from build123d import *

# Parameters (mm, degrees)
SKETCH1_R             = 30.5
SKETCH1_R_2           = 28.5
BOSS_EXTRUDE1_DEPTH   = 1.3
BOSS_EXTRUDE1_2_DEPTH = 1.3
BOSS_EXTRUDE1_3_DEPTH = 1.3
BOSS_EXTRUDE1_4_DEPTH = 1.3
SKETCH3_R             = 1
BOSS_EXTRUDE2_DEPTH   = 1.3


with BuildPart() as part:
    # Sketch1 → Boss-Extrude1 (new body)
    with BuildSketch(Plane.XY):
        with Locations((-31.819805153, 31.819805153)):
            Circle(SKETCH1_R)
        with Locations((-31.819805153, 31.819805153)):
            Circle(SKETCH1_R_2, mode=Mode.SUBTRACT)
    extrude(amount=BOSS_EXTRUDE1_DEPTH)



with BuildPart() as body_2:
    # Sketch1 → Boss-Extrude1 2 (new body)
    with BuildSketch(Plane.XY):
        with Locations((31.819805153, 31.819805153)):
            Circle(SKETCH1_R)
        with Locations((31.819805153, 31.819805153)):
            Circle(SKETCH1_R_2, mode=Mode.SUBTRACT)
    extrude(amount=BOSS_EXTRUDE1_2_DEPTH)


with BuildPart() as body_3:
    # Sketch1 → Boss-Extrude1 3 (new body)
    with BuildSketch(Plane.XY):
        with Locations((31.819805153, -31.819805153)):
            Circle(SKETCH1_R)
        with Locations((31.819805153, -31.819805153)):
            Circle(SKETCH1_R_2, mode=Mode.SUBTRACT)
    extrude(amount=BOSS_EXTRUDE1_3_DEPTH)


with BuildPart() as body_4:
    # Sketch1 → Boss-Extrude1 4 (new body)
    with BuildSketch(Plane.XY):
        with Locations((-31.819805153, -31.819805153)):
            Circle(SKETCH1_R)
        with Locations((-31.819805153, -31.819805153)):
            Circle(SKETCH1_R_2, mode=Mode.SUBTRACT)
    extrude(amount=BOSS_EXTRUDE1_4_DEPTH)


with BuildPart() as part_1:
    add(part.part)

    add(body_2.part)  # Boss-Extrude2 merges body 2

    add(body_3.part)  # Boss-Extrude2 merges body 3

    add(body_4.part)  # Boss-Extrude2 merges body 4
    # Sketch3 → Boss-Extrude2 (add)
    with BuildSketch(Plane(origin=(0, 0, 0), x_dir=(-1, 0, 0), z_dir=(0, 0, -1))):
        with BuildLine():
            ThreePointArc((-23.75, 0), (-20.75, -3), (-17.75, 0))
            ThreePointArc((-17.75, 0), (-20.75, 3), (-23.75, 0))
        make_face()
        with Locations((-20.75, 0)):
            Circle(SKETCH3_R, mode=Mode.SUBTRACT)
        with BuildLine():
            ThreePointArc((-14.160081763, -6.952473777), (-16.799552066, -3.912301259), (-17.75, 0))
            ThreePointArc((-17.75, 0), (-20.75, -3), (-23.75, 0))
            ThreePointArc((-23.75, 0), (-24.444680466, -1.473679275), (-26.023521849, -1.875638779))
            ThreePointArc((-26.023521849, -1.875638779), (-19.820237414, -3.779470382), (-14.160081763, -6.952473777))
        make_face()
        with BuildLine():
            ThreePointArc((-23.75, 0), (-20.75, 3), (-17.75, 0))
            ThreePointArc((-17.75, 0), (-16.799552066, 3.912301259), (-14.160081763, 6.952473777))
            ThreePointArc((-14.160081763, 6.952473777), (-19.820237414, 3.779470382), (-26.023521849, 1.875638779))
            ThreePointArc((-26.023521849, 1.875638779), (-24.444680466, 1.473679275), (-23.75, 0))
        make_face()
        with BuildLine():
            add(Edge.make_bspline(
                [(-14.160081763, -6.952473777), (-14.006442935, -7.061581552), (-11.281305453, -8.851296282), (-5.533016891, -10.311083757), (-0.273902085, -10.375), (0, -10.375)],
                knots=[0, 0, 0, 0, 0.05, 0.95, 1, 1, 1, 1], degree=3))
            ThreePointArc((-14.160081763, -6.952473777), (-7.656423025, -13.208492354), (-3.268059498, -21.093770469))
            ThreePointArc((-3.268059498, -21.093770469), (-2.8699742, -17.878412259), (0, -16.375))
            ThreePointArc((0, -16.375), (-3, -13.375), (0, -10.375))
        make_face()
        with BuildLine():
            ThreePointArc((-3.268059498, 21.093770469), (-7.656423025, 13.208492354), (-14.160081763, 6.952473777))
            add(Edge.make_bspline(
                [(-14.160081763, 6.952473777), (-14.006442935, 7.061581552), (-11.281305453, 8.851296282), (-5.533016891, 10.311083757), (-0.273902085, 10.375), (0, 10.375)],
                knots=[0, 0, 0, 0, 0.05, 0.95, 1, 1, 1, 1], degree=3))
            ThreePointArc((0, 10.375), (-3, 13.375), (0, 16.375))
            ThreePointArc((0, 16.375), (-2.8699742, 17.878412259), (-3.268059498, 21.093770469))
        make_face()
        with BuildLine():
            add(Edge.make_bspline(
                [(14.160081763, -6.952473777), (14.006442935, -7.061581552), (11.281305453, -8.851296282), (5.533016891, -10.311083757), (0.273902085, -10.375), (0, -10.375)],
                knots=[0, 0, 0, 0, 0.05, 0.95, 1, 1, 1, 1], degree=3))
            ThreePointArc((0, -10.375), (2.121320344, -11.253679656), (3, -13.375))
            ThreePointArc((3, -13.375), (2.121320344, -15.496320344), (0, -16.375))
            ThreePointArc((0, -16.375), (2.8699742, -17.878412259), (3.268059498, -21.093770469))
            ThreePointArc((3.268059498, -21.093770469), (7.656423025, -13.208492354), (14.160081763, -6.952473777))
        make_face()
        with BuildLine():
            ThreePointArc((3, -13.375), (2.121320344, -11.253679656), (0, -10.375))
            ThreePointArc((0, -10.375), (-3, -13.375), (0, -16.375))
            ThreePointArc((0, -16.375), (2.121320344, -15.496320344), (3, -13.375))
        make_face()
        with Locations((0, -13.375)):
            Circle(SKETCH3_R, mode=Mode.SUBTRACT)
        with BuildLine():
            ThreePointArc((0, 16.375), (-3, 13.375), (0, 10.375))
            ThreePointArc((0, 10.375), (2.121320344, 11.253679656), (3, 13.375))
            ThreePointArc((3, 13.375), (2.121320344, 15.496320344), (0, 16.375))
        make_face()
        with Locations((0, 13.375)):
            Circle(SKETCH3_R, mode=Mode.SUBTRACT)
        with BuildLine():
            ThreePointArc((3, 13.375), (2.121320344, 11.253679656), (0, 10.375))
            add(Edge.make_bspline(
                [(14.160081763, 6.952473777), (14.006442935, 7.061581552), (11.281305453, 8.851296282), (5.533016891, 10.311083757), (0.273902085, 10.375), (0, 10.375)],
                knots=[0, 0, 0, 0, 0.05, 0.95, 1, 1, 1, 1], degree=3))
            ThreePointArc((14.160081763, 6.952473777), (7.656423025, 13.208492354), (3.268059498, 21.093770469))
            ThreePointArc((3.268059498, 21.093770469), (2.8699742, 17.878412259), (0, 16.375))
            ThreePointArc((0, 16.375), (2.121320344, 15.496320344), (3, 13.375))
        make_face()
        with BuildLine():
            ThreePointArc((17.75, 0), (16.799552066, -3.912301259), (14.160081763, -6.952473777))
            ThreePointArc((14.160081763, -6.952473777), (19.820237414, -3.779470382), (26.023521849, -1.875638779))
            ThreePointArc((26.023521849, -1.875638779), (24.444680466, -1.473679275), (23.75, 0))
            ThreePointArc((23.75, 0), (24.444680466, 1.473679275), (26.023521849, 1.875638779))
            ThreePointArc((26.023521849, 1.875638779), (19.820237414, 3.779470382), (14.160081763, 6.952473777))
            ThreePointArc((14.160081763, 6.952473777), (16.799552066, 3.912301259), (17.75, 0))
        make_face()
        with Locations((20.75, 0)):
            Circle(SKETCH3_R, mode=Mode.SUBTRACT)
        with Locations((20.75, 0)):
            Circle(SKETCH3_R)
    extrude(amount=-BOSS_EXTRUDE2_DEPTH)


solid = part_1.part
Model file for the job. Use its own axes, mm. Coordinates: 2 decimals unless noted, no trailing zeros. Order: outer loops, then holes, each group sorted by start corner. A loop starts at its lowest first (then second) coordinate and runs counter-clockwise, first axis right, second up. Notation, with made-up numbers: (23.25, 23) -> (42.25, 23) arc R8 ccw to (42.25, 33) -> close; hole circle Ø3 at (70.25, 39.5). An arc over 180 degrees is marked (long way). Return JSON: item names as keys, results as strings. Group by question number.
Item 1: Saw through at A-A on y = 23. Write the cut outline in (x, z), then the cut area to 3 significant figures.
Item 2: Pull direction X, two halves, no side cores. Call faces 1 (the cylindrical face through (-54.44, 14.48, 0.64)), 2 (the flat face through (10, 10, 1.3)): pulls with the +X half, pulls with the -X half, needs draft (parallel to the pull), parting line crosses it, or undercut.
Item 3: Saw through at B-B on y = -48. Write the cut outline in (x, z).
Item 4: Saw through at C-C on z = 0.25. State how many separate pieces and enclosed holes the cut face has, then the cut area to 3 significant figures.
Item 5: Wall check: line 1 along X through (y, z) = (-31.5, 1.1); line 2 along Y through (x, z) = (53, 0.4); line 3 along Y through (x, z) = (-29.5, 0.9). Give the ranges that are in metal, low to high. Write a range as [from, to].
Values found:
{
 "1": {"outline": "(-61.02, 0) -> (-58.92, 0) -> (-58.92, 1.3) -> (-61.02, 1.3) -> close; (-4.72, 0) -> (-2.62, 0) -> (-2.62, 1.3) -> (-4.72, 1.3) -> close; (2.62, 0) -> (4.72, 0) -> (4.72, 1.3) -> (2.62, 1.3) -> close; (58.92, 0) -> (61.02, 0) -> (61.02, 1.3) -> (58.92, 1.3) -> close", "area": "10.9 mm2"},
 "2": {"face 1": "undercut", "face 2": "needs draft"},
 "3": {"outline": "(-57.67, 0) -> (-55.28, 0) -> (-55.28, 1.3) -> (-57.67, 1.3) -> close; (-8.36, 0) -> (-5.97, 0) -> (-5.97, 1.3) -> (-8.36, 1.3) -> close; (5.97, 0) -> (8.36, 0) -> (8.36, 1.3) -> (5.97, 1.3) -> close; (55.28, 0) -> (57.67, 0) -> (57.67, 1.3) -> (55.28, 1.3) -> close"},
 "4": {"separate pieces": "1", "enclosed holes": "8", "area": "1,810 mm2"},
 "5": {"line 1": "x = [-62.32, -60.32], [-3.32, -1.32], [1.32, 3.32], [60.32, 62.32]", "line 2": "y = [-53.77, -50.89], [-12.75, -9.87], [9.87, 12.75], [50.89, 53.77]", "line 3": "y = [-62.23, -60.23], [-3.41, -1.41], [1.41, 3.41], [60.23, 62.23]"}
}
